Design review of the part built by this model. Coordinates are the model's own, in mm. Face numbers are marked on the shaded views. A direction names the side the tool comes from. Coordinates: 2 decimals unless noted, no trailing zeros. Order: outer loops, then holes, each group sorted by start corner. A loop starts at its lowest first (then second) coordinate and runs counter-clockwise, first axis right, second up. Notation, with made-up numbers: (15.25, -12.75) -> (19.25, -12.75) arc R26 ccw to (19.25, 25.25) -> close; hole circle Ø9 at (53.5, 86.25). An arc over 180 degrees is marked (long way). Write item = value, one per line.
```python
from build123d import *

# Parameters (mm, degrees)
F0_W     = 12.7
F0_H     = 50.8
F1_DEPTH = 3.175
F2_R     = 4.7625
F3_DEPTH = 3.175
F5_DEPTH = 3.175


with BuildPart() as f1:
    # F0 (on Top) → F1 (new body)
    with BuildSketch(Plane.XY):
        Rectangle(F0_W, F0_H)
    extrude(amount=F1_DEPTH)

    # F2 (on face) → F3 (cut, through all)
    with BuildSketch(Plane.XY.offset(3.175)):
        with Locations((0, 12.7)):
            Circle(F2_R)
    extrude(amount=-F3_DEPTH, mode=Mode.SUBTRACT)

    # F4 (on face) → F5 (cut, through all)
    with BuildSketch(Plane.XY.offset(3.175)):
        with BuildLine():
            Line((1.4605, 25.4), (-1.7145, 25.4))
            Line((-1.7145, 25.4), (-1.7145, 17.233028))
            Line((-1.7145, 17.233028), (-1.4605, 17.233028))
            ThreePointArc((-1.4605, 17.233028), (0, 17.4625), (1.4605, 17.233028))
            Line((1.4605, 17.233028), (1.4605, 25.4))
        make_face()
    extrude(amount=-F5_DEPTH, mode=Mode.SUBTRACT)


solid = f1.part
```
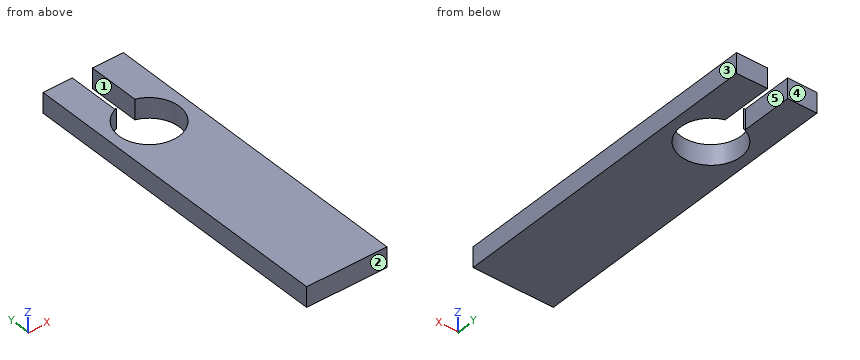
(1) For the marked faces 4 and 5, list the 3-axis set-ups (+Z, -Z, +X, -X, +Y, -Y) from which the entire face can be reached by the end or side of a thin tool; tool diameter is ignored.
Report:
face_4 = +Z, -Z, +X, -X, +Y
face_5 = +Z, -Z, +Y
(2) We need section B-B (x = 2.75). Write out the cut boundary in (y, z) (3 decimals), and give its area (3 significant figures).
Report:
outline = (-25.4, 0) -> (8.812, 0) -> (8.812, 3.175) -> (-25.4, 3.175) -> close; (16.588, 0) -> (25.4, 0) -> (25.4, 3.175) -> (16.588, 3.175) -> close
area = 137 mm²
(3) We need section D-D (x = 0). Write out the cut boundary in (y, z) (1 decimal), and give its area (3 significant figures).
Report:
outline = (-25.4, 0) -> (7.9, 0) -> (7.9, 3.2) -> (-25.4, 3.2) -> close
area = 106 mm²
(4) The part is to be moulded in two halves that separate along X. For the marked faces 1, 2 and 3, say which applies: released by +X, released by -X, zero draft, split by the parting line, or undercut.
Report:
face_1 = undercut
face_2 = zero draft
face_3 = released by +X
(5) For L1, parallel to X at y = 12.7, z = 1.4; L2, parallel to Y at x = 0, z = 1.85; L3, parallel to X at y = 14, z = 1.9, list the stretches that pass through material, from the lowest coordinate up.
Report:
L1 = -6.35 to -4.76, 4.76 to 6.35
L2 = -25.4 to 7.94
L3 = -6.35 to -4.58, 4.58 to 6.35
